from build123d import *

# Parameters (mm, degrees)
SKETCH_1_R      = 31.75
EXTRUDE_2_DEPTH = 20
EXTRUDE_5_DEPTH = 20.5
FILLET_1_R      = 3


with BuildPart() as part:
    # 草图1 → 凸台-拉伸2 (new body)
    with BuildSketch(Plane(origin=(0, 0, 0), x_dir=(1, 0, 0), z_dir=(0, 1, 0))):
        with Locations(Location((0, 0, 0), (0, 0, 270))):
            Circle(SKETCH_1_R)
    extrude(amount=EXTRUDE_2_DEPTH)

    # 草图3 → 凸台-拉伸5 (add)
    with BuildSketch(Plane.XZ):
        with BuildLine():
            Line((46.5, 18.914280319), (10.725, 31.208562527))
            ThreePointArc((10.725, 31.208562527), (5.436793017, 32.549059613), (0, 33))
            ThreePointArc((0, 33), (-14.61315827, 31.767511075), (-28.813455811, 28.1048654))
            ThreePointArc((-28.813455811, 28.1048654), (-33, 0), (-28.813455811, -28.1048654))
            ThreePointArc((-28.813455811, -28.1048654), (-14.61315827, -31.767511075), (0, -33))
            ThreePointArc((0, -33), (6.028677808, -32.444645843), (11.854443416, -30.797275387))
            Line((11.854443416, -30.797275387), (44.146384059, -19.565467008))
            ThreePointArc((44.146384059, -19.565467008), (59.962693004, -1.221019257), (46.5, 18.914280319))
        make_face()
    extrude(amount=EXTRUDE_5_DEPTH)

    # 圆角1
    fillet_1_edges = [part.edges().sort_by_distance(p)[0] for p in [
        (-28.813455811, -10.25, 28.1048654),
        (-28.813455811, -10.25, -28.1048654),
    ]]
    fillet(fillet_1_edges, radius=FILLET_1_R)


solid = part.part
The listing builds one solid part. Answer for the finished solid, in the listing's coordinates (mm). A direction names the side the tool comes from. Give positions to 0.01 mm unless a question says otherwise; leave off trailing zeros. Write each loop counter-clockwise with the first axis right and the second up, starting at its lowest first coordinate (ties: lowest second). Pieces come first, ordered by that corner, then holes. Notation, with made-up numbers: (45, 50) - (65, 50) arc R23 cw to (65, 60) - close; hole circle Ø11 at (77.25, 18.5). An arc over 180 degrees is marked (long way). Use a Markdown table: item, result.
1. A tool of negligible diameter and unlimited length cuts with its end or side. For faces 1 (the flat face through (34, 0, 3)), 2 (the cylindrical face through (5.512, -10.106, 32.536)), from which of +Z, -Z, +X, -X, +Y, -Y can it reach the whole face along a straight path? Write none if from no direction.
Values follow:
| item | result |
|---|---|
| face 1 | +Y |
| face 2 | +Z, +X, +Y, -Y |
2. Section D-D on x = 53.5 is taken. Write down the section's boundary in (y, z).
Values follow:
| item | result |
|---|---|
| outline | (-20.5, -14.76) - (0, -14.76) - (0, 14.76) - (-20.5, 14.76) - close |
3. Each of these flat-tipped pins is pushed along its axis until it touches: P1, Ø3, axis at y = 6.5, z = 6, coming from the +X side; P2, Ø3, axis at y = 15.5, z = -18.5, coming from the -X side; P3, Ø1, axis at y = -1.5, z = -1.5, coming from the +X side (3 decimals). Where does it stop, or does it pass through?
Values follow:
| item | result |
|---|---|
| P1 | stops at x = 31.43 |
| P2 | stops at x = -26.82 |
| P3 | stops at x = 59.975 |
4. Section C-C on y = 13.5 is taken. Write down the section's boundary in (x, z).
Values follow:
| item | result |
|---|---|
| outline | circle Ø63.5 at (0, 0) |
5. Section A-A on z = 0 is taken. Write down the section's boundary in (x, y).
Values follow:
| item | result |
|---|---|
| outline | (-33, -20.5) - (60, -20.5) - (60, 0) - (31.75, 0) - (31.75, 20) - (-31.75, 20) - (-31.75, 0) - (-33, 0) - close |
6. Find the intervals of material crossed by probe 1 along Z at (x, y) = (-1.5, -17); probe 2 along Y at (x, z) = (51.5, 14); probe 3 along Z at (x, y) = (-6, -6), in increasing order. Write a range as from..to.
Values follow:
| item | result |
|---|---|
| probe 1 | z = -32.99..32.99 |
| probe 2 | y = -20.5..0 |
| probe 3 | z = -32.79..32.79 |
7. Section B-B on x = -6 is taken. Write down the section's boundary in (y, z).
Values follow:
| item | result |
|---|---|
| outline | (-20.5, -32.79) - (0, -32.79) - (0, -31.18) - (20, -31.18) - (20, 31.18) - (0, 31.18) - (0, 32.79) - (-20.5, 32.79) - close |
